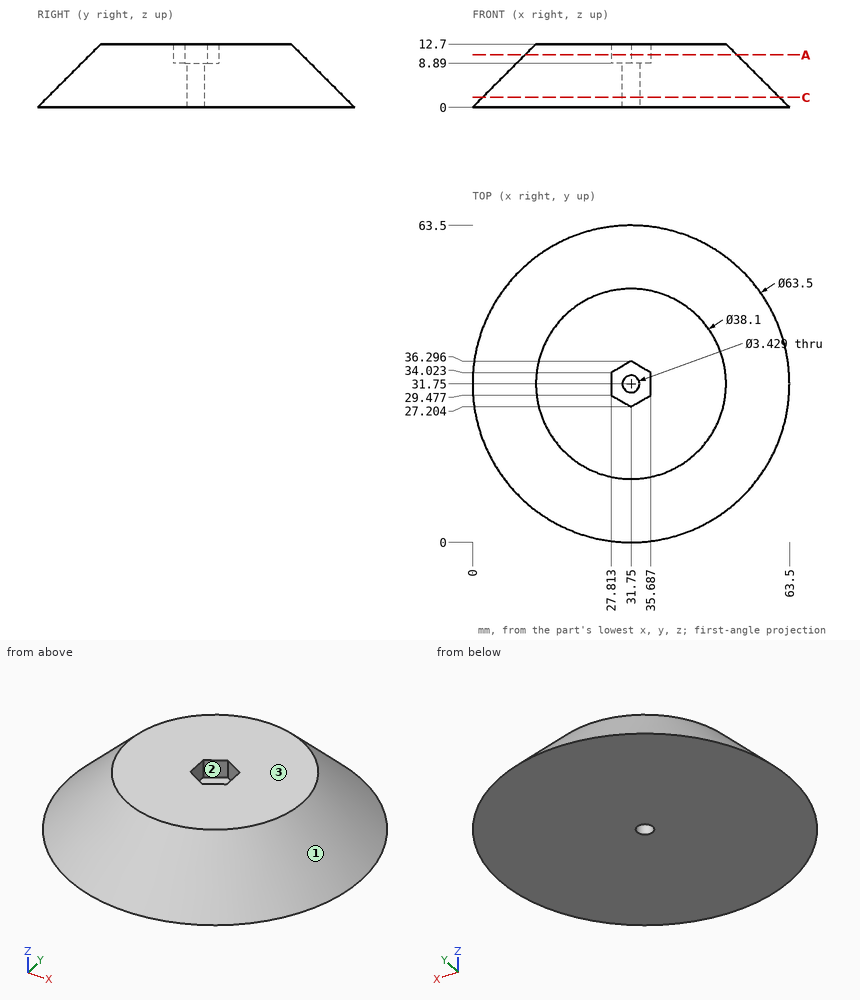
Check sheet for the drawn part. Datum: minimum x, y, z corner. Units: mm. Give positions to 0.01 mm unless a question says otherwise; leave off trailing zeros. Write each loop counter-clockwise with the first axis right and the second up, starting at its lowest first coordinate (ties: lowest second). Pieces come first, ordered by that corner, then holes.
(1) Mould release check, pull along Y, two halves, no side actions. Record for the marked faces 1, 2 and 3: +Y half, -Y half, draft (parallel to the pull), parting line (faces both ways), or undercut.
(2) Cross-section at A-A (z = 10.5). Enter the section's corners in (x, y), plus the area to 3 significant figures.
(3) Material ranges on line 1 (X direction, y = 33, z = 2.25); line 2 (Y direction, x = 31.75, z = 4); line 3 (Y direction, x = 31.75, z = 7.25), recorded low to high.
(4) Gauge pin test, flat ends, axial feed: pin 1 (1.5 mm diameter, centred on y = 8, z = 11, fed in from -X); pin 2 (2.5 mm diameter, centred on x = 33.5, y = 32, fed in from +Z); pin 3 (4 mm diameter, centred on x = 51, z = 7, fed in from -Y); pin 4 (5 mm diameter, centred on x = 39.5, z = 4, fed in from -Y). Record the tip position at first contact, or that the pin passes through.
(5) Cross-section at C-C (z = 2). Enter the section's corners in (x, y), plus the area to 3 significant figures.
Worked out:
1. face 1: parting line
1. face 2: undercut
1. face 3: draft
2. outline: circle Ø42.5 at (31.75, 31.75); hole (27.81, 29.48) - (31.75, 27.2) - (35.69, 29.48) - (35.69, 34.02) - (31.75, 36.3) - (27.81, 34.02) - close
2. area: 1,360 mm2
3. line 1: x = 2.28 to 30.58, 32.92 to 61.22
3. line 2: y = 4 to 30.04, 33.46 to 59.5
3. line 3: y = 7.25 to 30.04, 33.46 to 56.25
4. pin 1: passes through
4. pin 2: stops at z = 8.89
4. pin 3: stops at y = 12.55
4. pin 4: stops at y = 2.43
5. outline: circle Ø59.5 at (31.75, 31.75); hole circle Ø3.43 at (31.75, 31.75)
5. area: 2,770 mm2
